The listing builds one solid part. Answer for the finished solid, in the listing's coordinates (mm). A direction names the side the tool comes from. Coordinates: 2 decimals unless noted, no trailing zeros. Loops run counter-clockwise (first coordinate to the right, second up) from the corner with the lowest first, then second, coordinate; pieces in that order, holes last. Notation, with made-up numbers: (22.25, 40) - (58.25, 40) arc R20 cw to (58.25, 52) - close; hole circle Ø8 at (41.5, 32). An arc over 180 degrees is marked (long way). One line per question, with ' | ' between items.
from build123d import *
from OCP.BRepFilletAPI import BRepFilletAPI_MakeChamfer

# Parameters (mm, degrees)
SALIENTE_EXTRUIR1_DEPTH      = 2.5
REDONDEO1_R                  = 10
REDONDEO2_R                  = 30
REDONDEO3_R                  = 5
REDONDEO4_R                  = 2
CROQUIS2_R                   = 1.25
CORTAR_EXTRUIR1_DEPTH        = 2.5
CROQUIS3_W                   = 30
CROQUIS3_H                   = 2
SALIENTE_EXTRUIR2_DEPTH      = 3
CROQUIS4_R                   = 1
CROQUIS4_R_2                 = 1.25
CORTAR_EXTRUIR2_DEPTH        = 2.5
CROQUIS5_R                   = 1.25
CORTAR_EXTRUIR3_DEPTH        = 2.5
CROQUIS6_W                   = 30
CROQUIS6_H                   = 2
SALIENTE_EXTRUIR3_DEPTH      = 3
REDONDEO5_R                  = 1
SALIENTE_EXTRUIR6_DEPTH      = 2.5
REDONDEO7_R                  = 10
REDONDEO8_R                  = 3
CROQUIS8_W                   = 89
CROQUIS8_H                   = 6
CORTAR_EXTRUIR5_DEPTH        = 2.5
REDONDEO10_R                 = 1
CROQUIS9_W                   = 2.5
CROQUIS9_H                   = 5
SALIENTE_EXTRUIR7_DEPTH      = 5
REDONDEO11_R                 = 2.5
CROQUIS10_W                  = 1.5
CROQUIS10_H                  = 5
CORTAR_EXTRUIR6_DEPTH        = 2.5
CHAFL_N1_SIZE2               = 2.5
CHAFL_N1_SIZE                = 1.165769145
CROQUIS11_W                  = 2.5
CROQUIS11_H                  = 5
SALIENTE_EXTRUIR8_DEPTH      = 5
CROQUIS12_W                  = 1.25
CROQUIS12_H                  = 5
CORTAR_EXTRUIR7_DEPTH        = 2.5
CHAFL_N2_SIZE2               = 1.165769145
CHAFL_N2_SIZE                = 2.5
REDONDEO13_R                 = 2.5
CROQUIS13_W                  = 5
CROQUIS13_H                  = 2.5
SALIENTE_EXTRUIR9_DEPTH      = 5
REDONDEO14_R                 = 2.5
CROQUIS14_W                  = 5
CROQUIS14_H                  = 1.25
CORTAR_EXTRUIR8_DEPTH        = 2.5
CHAFL_N3_SIZE                = 1.165769145
CHAFL_N3_SIZE_2              = 2.5
REDONDEO14_OF_SIMETR_A4_R    = 2.5
CHAFL_N3_OF_SIMETR_A4_SIZE   = 1.165769145
CHAFL_N3_OF_SIMETR_A4_SIZE_2 = 2.5
CROQUIS17_W                  = 10
CROQUIS17_H                  = 40
CORTAR_EXTRUIR9_DEPTH        = 2.5
REDONDEO19_R                 = 5


with BuildPart() as part:
    # Croquis1 → Saliente-Extruir1 (new body)
    with BuildSketch(Plane.XY):
        Polygon((10, 22.5), (10, 65.5), (-10, 65.5), (-10, 22.5), (-50, 22.5), (-50, -2.5), (-67, -2.5), (-67, -36.5), (-50, -36.5), (-50, -65.5), (50, -65.5), (50, -36.5), (67, -36.5), (67, -2.5), (50, -2.5), (50, 22.5), align=None)
    extrude(amount=SALIENTE_EXTRUIR1_DEPTH)

    # Redondeo1
    redondeo1_edges = [part.edges().sort_by_distance(p)[0] for p in [
        (-50, -36.5, 1.25),
        (-50, -2.5, 1.25),
        (-50, 22.5, 1.25),
        (50, 22.5, 1.25),
        (50, -2.5, 1.25),
        (50, -36.5, 1.25),
    ]]
    fillet(redondeo1_edges, radius=REDONDEO1_R)

    # Redondeo2
    redondeo2_edges = [part.edges().sort_by_distance(p)[0] for p in [
        (10, 22.5, 1.25),
        (-10, 22.5, 1.25),
    ]]
    fillet(redondeo2_edges, radius=REDONDEO2_R - 0.0001)  # a hair under: the kernel refuses the full size

    # Redondeo3
    redondeo3_edges = [part.edges().sort_by_distance(p)[0] for p in [
        (50, -65.5, 1.25),
        (-50, -65.5, 1.25),
    ]]
    fillet(redondeo3_edges, radius=REDONDEO3_R)

    # Redondeo4
    redondeo4_edges = [part.edges().sort_by_distance(p)[0] for p in [
        (-67, -36.5, 1.25),
        (-67, -2.5, 1.25),
        (67, -2.5, 1.25),
        (67, -36.5, 1.25),
    ]]
    fillet(redondeo4_edges, radius=REDONDEO4_R)

    # Croquis2 → Cortar-Extruir1 (cut)
    with BuildSketch(Plane(origin=(0, 0, 0), x_dir=(-1, 0, 0), z_dir=(0, 0, -1))):
        with Locations((-15.7, -51.32)):
            Circle(CROQUIS2_R)
    cortar_extruir1 = extrude(amount=-CORTAR_EXTRUIR1_DEPTH, mode=Mode.SUBTRACT)

    # Simetría1: Cortar-Extruir1 across plane
    add(cortar_extruir1.mirror(Plane(origin=(0, 0, 0), x_dir=(0, 0, 1), z_dir=(1, 0, 0))), mode=Mode.SUBTRACT)

    # Croquis3 → Saliente-Extruir2 (add)
    with BuildSketch(Plane.XY.offset(2.5)):
        with Locations((0, -41)):
            Rectangle(CROQUIS3_W, CROQUIS3_H)
    extrude(amount=SALIENTE_EXTRUIR2_DEPTH)

    # Croquis4 → Cortar-Extruir2 (cut)
    with BuildSketch(Plane.XY.offset(2.5)):
        with Locations((64.5, -28.5)):
            Circle(CROQUIS4_R)
        with Locations((64.5, -10.5)):
            Circle(CROQUIS4_R)
        with Locations((41.5, -28.5)):
            Circle(CROQUIS4_R)
        with Locations((41.5, -10.5)):
            Circle(CROQUIS4_R)
        with Locations((0, -9.5)):
            Circle(CROQUIS4_R_2)
        with Locations((0, -29.5)):
            Circle(CROQUIS4_R_2)
    cortar_extruir2 = extrude(amount=-CORTAR_EXTRUIR2_DEPTH, mode=Mode.SUBTRACT)

    # Simetría2: Cortar-Extruir2 across plane
    add(cortar_extruir2.mirror(Plane(origin=(0, 0, 0), x_dir=(0, 0, 1), z_dir=(1, 0, 0))), mode=Mode.SUBTRACT)

    # Croquis5 → Cortar-Extruir3 (cut)
    with BuildSketch(Plane.XY.offset(2.5)):
        with Locations((38.2, 8.5)):
            Circle(CROQUIS5_R)
    cortar_extruir3 = extrude(amount=-CORTAR_EXTRUIR3_DEPTH, mode=Mode.SUBTRACT)

    # Simetría3: Cortar-Extruir3 across plane
    add(cortar_extruir3.mirror(Plane(origin=(0, 0, 0), x_dir=(0, 0, 1), z_dir=(1, 0, 0))), mode=Mode.SUBTRACT)

    # Croquis6 → Saliente-Extruir3 (add)
    with BuildSketch(Plane.XY.offset(2.5)):
        with Locations((0, 3)):
            Rectangle(CROQUIS6_W, CROQUIS6_H)
    extrude(amount=SALIENTE_EXTRUIR3_DEPTH)

    # Redondeo5
    redondeo5_edges = [part.edges().sort_by_distance(p)[0] for p in [
        (-15, -41, 2.5),
        (0, -42, 2.5),
        (15, -41, 2.5),
        (-15, 3, 2.5),
        (15, 3, 2.5),
        (0, 4, 2.5),
    ]]
    fillet(redondeo5_edges, radius=REDONDEO5_R)

    # Croquis7 → Saliente-Extruir6 (add)
    with BuildSketch(Plane.XY.offset(2.5)):
        Polygon((10, 65.5), (10, 76.5), (57.5, 76.5), (57.5, 101.5), (-54.5, 101.5), (-54.5, 76.5), (-10, 76.5), (-10, 65.5), align=None)
    extrude(amount=-SALIENTE_EXTRUIR6_DEPTH)

    # Redondeo7
    redondeo7_edges = [part.edges().sort_by_distance(p)[0] for p in [
        (10, 76.5, 1.25),
        (-10, 76.5, 1.25),
    ]]
    fillet(redondeo7_edges, radius=REDONDEO7_R)

    # Redondeo8
    redondeo8_edges = [part.edges().sort_by_distance(p)[0] for p in [
        (-54.5, 76.5, 1.25),
        (-54.5, 101.5, 1.25),
        (57.5, 101.5, 1.25),
        (57.5, 76.5, 1.25),
    ]]
    fillet(redondeo8_edges, radius=REDONDEO8_R)

    # Croquis8 → Cortar-Extruir5 (cut)
    with BuildSketch(Plane.XY.offset(2.5)):
        with Locations((0, 86.5)):
            Rectangle(CROQUIS8_W, CROQUIS8_H)
    extrude(amount=-CORTAR_EXTRUIR5_DEPTH, mode=Mode.SUBTRACT)

    # Redondeo10
    redondeo10_edges = [part.edges().sort_by_distance(p)[0] for p in [
        (-44.5, 83.5, 1.25),
        (-44.5, 89.5, 1.25),
        (44.5, 89.5, 1.25),
        (44.5, 83.5, 1.25),
    ]]
    fillet(redondeo10_edges, radius=REDONDEO10_R)

    # Croquis9 → Saliente-Extruir7 (add)
    with BuildSketch(Plane.XY.offset(2.5)):
        with Locations((-50.75, 87.094539416)):
            Rectangle(CROQUIS9_W, CROQUIS9_H)
    extrude(amount=SALIENTE_EXTRUIR7_DEPTH)

    # Redondeo11
    redondeo11_edges = [part.edges().sort_by_distance(p)[0] for p in [
        (-52, 87.094539416, 2.5),
    ]]
    fillet(redondeo11_edges, radius=REDONDEO11_R - 0.0001)  # a hair under: the kernel refuses the full size

    # Croquis10 → Cortar-Extruir6 (cut)
    with BuildSketch(Plane.XY.offset(2.5)):
        with Locations((-50.25, 87.094539416)):
            Rectangle(CROQUIS10_W, CROQUIS10_H)
    extrude(amount=CORTAR_EXTRUIR6_DEPTH, mode=Mode.SUBTRACT)

    # Chaflán1
    chafl_n1_edges = [part.edges().sort_by_distance(p)[0] for p in [
        (-49.5, 87.094539416, 7.5),
    ]]
    chafl_n1_side = [part.faces().sort_by_distance(p)[0] for p in [
        (-49.523315383, 87.094539416, 7.5),
    ]]
    chamfer(chafl_n1_edges, length=CHAFL_N1_SIZE - 0.0001, length2=CHAFL_N1_SIZE2 - 0.0001, reference=chafl_n1_side[0])  # a hair under: the kernel refuses the full size

    # Croquis11 → Saliente-Extruir8 (add)
    with BuildSketch(Plane.XY.offset(2.5)):
        with Locations((53.75, 86.5)):
            Rectangle(CROQUIS11_W, CROQUIS11_H)
    extrude(amount=SALIENTE_EXTRUIR8_DEPTH)

    # Croquis12 → Cortar-Extruir7 (cut)
    with BuildSketch(Plane.XY.offset(2.5)):
        with Locations((53.125, 86.5)):
            Rectangle(CROQUIS12_W, CROQUIS12_H)
    extrude(amount=CORTAR_EXTRUIR7_DEPTH, mode=Mode.SUBTRACT)

    # Chaflán2
    chafl_n2_edges = [part.edges().sort_by_distance(p)[0] for p in [
        (52.5, 86.5, 7.5),
    ]]
    chafl_n2_side = [part.faces().sort_by_distance(p)[0] for p in [
        (52.5, 86.5, 7.476684617),
    ]]
    chamfer(chafl_n2_edges, length=CHAFL_N2_SIZE - 0.0001, length2=CHAFL_N2_SIZE2 - 0.0001, reference=chafl_n2_side[0])  # a hair under: the kernel refuses the full size

    # Redondeo13
    redondeo13_edges = [part.edges().sort_by_distance(p)[0] for p in [
        (55, 86.5, 2.5),
    ]]
    fillet(redondeo13_edges, radius=REDONDEO13_R - 0.0001)  # a hair under: the kernel refuses the full size

    # Croquis13 → Saliente-Extruir9 (add)
    with BuildSketch(Plane.XY.offset(2.5)):
        with Locations((-38.066978344, 97.75)):
            Rectangle(CROQUIS13_W, CROQUIS13_H)
        with Locations((-18.066978344, 97.75)):
            Rectangle(CROQUIS13_W, CROQUIS13_H)
    saliente_extruir9 = extrude(amount=SALIENTE_EXTRUIR9_DEPTH)

    # Redondeo14
    redondeo14_edges = [part.edges().sort_by_distance(p)[0] for p in [
        (-38.066978344, 99, 2.5),
        (-18.066978344, 99, 2.5),
    ]]
    fillet(redondeo14_edges, radius=REDONDEO14_R - 0.0001)  # a hair under: the kernel refuses the full size

    # Croquis14 → Cortar-Extruir8 (cut)
    with BuildSketch(Plane.XY.offset(2.5)):
        with Locations((-38.066978344, 97.125)):
            Rectangle(CROQUIS14_W, CROQUIS14_H)
        with Locations((-18.066978344, 97.125)):
            Rectangle(CROQUIS14_W, CROQUIS14_H)
    cortar_extruir8 = extrude(amount=CORTAR_EXTRUIR8_DEPTH, mode=Mode.SUBTRACT)

    # Chaflán3
    chafl_n3_edges_1 = [part.edges().sort_by_distance(p)[0] for p in [
        (-18.066978344, 96.5, 7.5),
    ]]
    chafl_n3_side_1 = [part.faces().sort_by_distance(p)[0] for p in [
        (-18.066978344, 96.523315383, 7.5),
    ]]
    chafl_n3_edges_2 = [part.edges().sort_by_distance(p)[0] for p in [
        (-38.066978344, 96.5, 7.5),
    ]]
    chafl_n3_side_2 = [part.faces().sort_by_distance(p)[0] for p in [
        (-38.066978344, 96.523315383, 7.5),
    ]]
    chafl_n3 = BRepFilletAPI_MakeChamfer(part.part.solid().wrapped)
    for e in chafl_n3_edges_1:
        chafl_n3.Add(CHAFL_N3_SIZE - 0.0001, CHAFL_N3_SIZE_2 - 0.0001, e.wrapped, chafl_n3_side_1[0].wrapped)
    for e in chafl_n3_edges_2:
        chafl_n3.Add(CHAFL_N3_SIZE - 0.0001, CHAFL_N3_SIZE_2 - 0.0001, e.wrapped, chafl_n3_side_2[0].wrapped)
    add(Compound.cast(chafl_n3.Shape()), mode=Mode.REPLACE)  # a hair under: the kernel refuses the full size

    # Simetría4: Saliente-Extruir9, Cortar-Extruir8 across plane
    add(saliente_extruir9.mirror(Plane(origin=(0, 0, 0), x_dir=(0, 0, 1), z_dir=(1, 0, 0))))
    add(cortar_extruir8.mirror(Plane(origin=(0, 0, 0), x_dir=(0, 0, 1), z_dir=(1, 0, 0))), mode=Mode.SUBTRACT)

    # Redondeo14 of Simetría4
    redondeo14_of_simetr_a4_edges = [part.edges().sort_by_distance(p)[0] for p in [
        (38.066978344, 99, 2.5),
        (18.066978344, 99, 2.5),
    ]]
    fillet(redondeo14_of_simetr_a4_edges, radius=REDONDEO14_OF_SIMETR_A4_R - 0.0001)  # a hair under: the kernel refuses the full size

    # Chaflán3 of Simetría4
    chafl_n3_of_simetr_a4_edges_1 = [part.edges().sort_by_distance(p)[0] for p in [
        (18.066978344, 96.5, 7.5),
    ]]
    chafl_n3_of_simetr_a4_side_1 = [part.faces().sort_by_distance(p)[0] for p in [
        (18.066978344, 96.523315383, 7.5),
    ]]
    chafl_n3_of_simetr_a4_edges_2 = [part.edges().sort_by_distance(p)[0] for p in [
        (38.066978344, 96.5, 7.5),
    ]]
    chafl_n3_of_simetr_a4_side_2 = [part.faces().sort_by_distance(p)[0] for p in [
        (38.066978344, 96.523315383, 7.5),
    ]]
    chafl_n3_of_simetr_a4 = BRepFilletAPI_MakeChamfer(part.part.solid().wrapped)
    for e in chafl_n3_of_simetr_a4_edges_1:
        chafl_n3_of_simetr_a4.Add(CHAFL_N3_OF_SIMETR_A4_SIZE - 0.0001, CHAFL_N3_OF_SIMETR_A4_SIZE_2 - 0.0001, e.wrapped, chafl_n3_of_simetr_a4_side_1[0].wrapped)
    for e in chafl_n3_of_simetr_a4_edges_2:
        chafl_n3_of_simetr_a4.Add(CHAFL_N3_OF_SIMETR_A4_SIZE - 0.0001, CHAFL_N3_OF_SIMETR_A4_SIZE_2 - 0.0001, e.wrapped, chafl_n3_of_simetr_a4_side_2[0].wrapped)
    add(Compound.cast(chafl_n3_of_simetr_a4.Shape()), mode=Mode.REPLACE)  # a hair under: the kernel refuses the full size

    # Croquis17 → Cortar-Extruir9 (cut)
    with BuildSketch(Plane.XY.offset(2.5)):
        with Locations((0, 44)):
            Rectangle(CROQUIS17_W, CROQUIS17_H)
    extrude(amount=-CORTAR_EXTRUIR9_DEPTH, mode=Mode.SUBTRACT)

    # Redondeo19
    redondeo19_edges = [part.edges().sort_by_distance(p)[0] for p in [
        (-5, 24, 1.25),
        (5, 24, 1.25),
        (5, 64, 1.25),
        (-5, 64, 1.25),
    ]]
    fillet(redondeo19_edges, radius=REDONDEO19_R - 0.0001)  # a hair under: the kernel refuses the full size


solid = part.part
Item 1: Each of these flat-tipped pins is pushed along its axis until it touches: pin 1 Ø1.2 at (y, z) = (86.5, 1.5) entering from +X; pin 2 Ø1 at (y, z) = (13.5, 2.5) entering from +X; pin 3 Ø3 at (x, z) = (-38.5, 4.5) entering from -Y. Where does it stop, or does it pass through?
Taken from the geometry:
pin 1: stops at x = 57.5 | pin 2: stops at x = 49.99 | pin 3: stops at y = 96.5
Item 2: Which of the six approach directions +Z, -Z, +X, -X, +Y, -Y give full straight-line access (tool end or side, diameter ignored) to faces 1 (the face through (-3, 63, 1)), 2 (the face through (-35.567, 98, 5)), 3 (the face through (54, 84, 5)), 4 (the face through (53.01, 0.35, 1.27)), 5 (the face through (-12.85, 73.49, 1.23))?
Taken from the geometry:
face 1: +Z, -Z | face 2: +Z, +Y, -Y | face 3: +Z, +X, -X, -Y | face 4: +Z, -Z, +X | face 5: +Z, -Z, -X
Item 3: Find section B-B, the plane y = -21.5. Write down the section's boundary in (x, z), plus the area to 3 significant figures.
Taken from the geometry:
outline: (-67, 0) - (67, 0) - (67, 2.5) - (-67, 2.5) - close | area: 335 mm2
Item 4: The mould has two halves that part along Y. Classify faces 6 (the face through (-51.5, 89.595, 4.8)), 7 (the face through (-52.85, 0.51, 1.27)), 8 (the face through (-40.567, 98, 5)): pulls with the +Y half, pulls with the -Y half, needs draft (parallel to the pull), parting line crosses it, or undercut.
Taken from the geometry:
face 6: pulls with the +Y half | face 7: undercut | face 8: needs draft
Item 5: Find section A-A, the plane y = 61. Write down the section's boundary in (x, z), plus the area to 3 significant figures.
Taken from the geometry:
outline: (-10, 0) - (-4.58, 0) - (-4.58, 2.5) - (-10, 2.5) - close; (4.58, 0) - (10, 0) - (10, 2.5) - (4.58, 2.5) - close | area: 27.1 mm2
Item 6: Find the intervals of material crossed by line 1 (Y direction, x = -64.5, z = 1.5); line 2 (Y direction, x = -38.2, z = 1.25); line 3 (Y direction, x = -43.5, z = 1), in increasing order. Write a range as [from, to].
Taken from the geometry:
line 1: y = [-36.5, -29.5], [-27.5, -11.5], [-9.5, -2.5] | line 2: y = [-65.5, 7.25], [9.75, 22.55], [76.5, 83.5], [89.5, 101.5] | line 3: y = [-65.5, 21.87], [76.5, 83.5], [89.5, 101.5]
